```python
from build123d import *

# Parameters (mm, degrees)
SKETCH1_W            = 101.6
SKETCH1_H            = 33.02
BOSS_EXTRUDE1_DEPTH  = 101.6
SKETCH2_W            = 63.5
SKETCH2_H            = 81.28
CUT_EXTRUDE1_DEPTH   = 119.294211186
BOSS_EXTRUDE2_START  = -16.51
BOSS_EXTRUDE2_DEPTH  = 3.81
FILLET2_R            = 2.54
SKETCH4_W            = 12.7
SKETCH4_H            = 12.7
SKETCH4_R            = 1.55
BOSS_EXTRUDE3_DEPTH  = 3.81
FILLET3_R            = 2.54
FILLET2_OF_MIRROR1_R = 2.54


with BuildPart() as part:
    # Sketch1 → Boss-Extrude1 (new body)
    with BuildSketch(Plane.XY):
        Rectangle(SKETCH1_W, SKETCH1_H)
        with BuildLine():
            Line((-31.75, 10.16), (31.75, 10.16))
            ThreePointArc((31.75, 10.16), (41.91, 0), (31.75, -10.16))
            Line((31.75, -10.16), (-31.75, -10.16))
            ThreePointArc((-31.75, -10.16), (-41.91, 0), (-31.75, 10.16))
        make_face(mode=Mode.SUBTRACT)
    extrude(amount=-BOSS_EXTRUDE1_DEPTH)

    # Sketch2 → Cut-Extrude1 (cut, through all)
    with BuildSketch(Plane(origin=(0, 16.51, 0), x_dir=(1, 0, 0), z_dir=(0, 1, 0))):
        with Locations((0, 50.8)):
            Rectangle(SKETCH2_W, SKETCH2_H)
    extrude(amount=-CUT_EXTRUDE1_DEPTH, mode=Mode.SUBTRACT)

    # Sketch3 → Boss-Extrude2 (add, symmetric)
    with BuildSketch(Plane(origin=(0, 16.51, 0), x_dir=(1, 0, 0), z_dir=(0, 1, 0)).offset(BOSS_EXTRUDE2_START)):
        Polygon((-42.926, -4.867948453), (-43.942, -7.195896906), (-42.926, -7.195896906), (-41.91, -4.867948453), (-40.894, -2.54), (-41.91, -2.54), (-41.91, 0), (-43.942, 0), align=None)
    boss_extrude2 = extrude(amount=BOSS_EXTRUDE2_DEPTH, both=True)

    # Fillet2
    fillet2_edges = [part.edges().sort_by_distance(p)[0] for p in [
        (-43.942, 0, 0),
    ]]
    fillet(fillet2_edges, radius=FILLET2_R)

    # Sketch4 → Boss-Extrude3 (add)
    # profile 1 of 4: a face of its own
    with BuildSketch(Plane.XZ.offset(16.51)):
        with Locations((-57.15, -95.25)):
            Rectangle(SKETCH4_W, SKETCH4_H)
        with Locations((-57.15, -95.25)):
            Circle(SKETCH4_R, mode=Mode.SUBTRACT)
    # profile 2 of 4: a face of its own
    with BuildSketch(Plane.XZ.offset(16.51)):
        with Locations((57.15, -95.25)):
            Rectangle(SKETCH4_W, SKETCH4_H)
        with Locations((57.15, -95.25)):
            Circle(SKETCH4_R, mode=Mode.SUBTRACT)
    # profile 3 of 4: a face of its own
    with BuildSketch(Plane.XZ.offset(16.51)):
        with Locations((57.15, -6.35)):
            Rectangle(SKETCH4_W, SKETCH4_H)
        with Locations((57.15, -6.35)):
            Circle(SKETCH4_R, mode=Mode.SUBTRACT)
    # profile 4 of 4: a face of its own
    with BuildSketch(Plane.XZ.offset(16.51)):
        with Locations((-57.15, -6.35)):
            Rectangle(SKETCH4_W, SKETCH4_H)
        with Locations((-57.15, -6.35)):
            Circle(SKETCH4_R, mode=Mode.SUBTRACT)
    extrude(amount=-BOSS_EXTRUDE3_DEPTH)

    # Fillet3
    fillet3_edges = [part.edges().sort_by_distance(p)[0] for p in [
        (-63.5, -12.7, -95.25),
        (-50.8, -12.7, -95.25),
        (63.5, -12.7, -95.25),
        (50.8, -12.7, -95.25),
        (63.5, -12.7, -6.35),
        (50.8, -12.7, -6.35),
        (-63.5, -12.7, -6.35),
        (-50.8, -12.7, -6.35),
    ]]
    fillet(fillet3_edges, radius=FILLET3_R)

    # Mirror1: Boss-Extrude2 across plane
    add(boss_extrude2.mirror(Plane(origin=(0, 0, 0), x_dir=(0, 0, 1), z_dir=(1, 0, 0))))

    # Fillet2 of Mirror1
    fillet2_of_mirror1_edges = [part.edges().sort_by_distance(p)[0] for p in [
        (43.942, 0, 0),
    ]]
    fillet(fillet2_of_mirror1_edges, radius=FILLET2_OF_MIRROR1_R)


solid = part.part
```
Source: CAD feature listing. Evaluate the final solid. Frame: model axes, mm. A direction names the side the tool comes from. Coordinates: 2 decimals unless noted, no trailing zeros. Order: outer loops, then holes, each group sorted by start corner. A loop starts at its lowest first (then second) coordinate and runs counter-clockwise, first axis right, second up. Notation, with made-up numbers: M -10.5,-39 L 10.5,-39 A14 ccw 10.5,-12 Z; hole C 31.25,88.5 d11. An arc over 180 degrees is marked long. Write each question's results on one line, items separated by ' | '. Start each with the question number.
1) Section query D-D (y = -2). Return the cut outline in (x, z).
2) Section query A-A (z = -67). Return the cut outline in (x, y), plus the area to 3 significant figures.
3) Line query: line 1 (Z direction, x = 57.15, y = -15.3); line 2 (X direction, y = -15, z = -95); line 3 (X direction, y = -14, z = -29). Output: solid intervals per line, ascending. Write a range as from..to.
4) Access query for faces 1 (the face through (50.8, 0, -50)), 2 (the face through (-57, -15, -88.9)), 3 (the face through (-50.8, 0, -50)), 4 (the face through (-58.1, -12.7, -4.8)), 5 (the face through (31.75, 13, -50)). Directions: +Z, -Z, +X, -X, +Y, -Y. A direction counts if a zero-diameter tool reaches every point of the face in a straight line with its end or side. Return the directions, or none.
5) Section query B-B (z = -6.35). Return the cut outline in (x, y).
6) Contact query for flat-ended pins moving along their axis: pin 1 Ø3 at (x, y) = (-54, -15) entering from +Z; pin 2 Ø1 at (y, z) = (5, -53) entering from +X; pin 3 Ø2.5 at (x, z) = (-43, 2) entering from -Y. Output: stop coordinate, or through.
7) Draft query along Z for faces 6 (the face through (41.924, 0.053, 4.901)), 7 (the face through (-43, 3.81, 3)), 8 (the face through (-1, -11, -101.6)), 9 (the face through (57, -15, -12.7)). Return one class per face: released by +Z, released by -Z, zero draft, split by the parting line, or undercut.
8) Section query C-C (x = 57.15). Return the cut outline in (y, z), plus the area to 3 significant figures.
Answers:
1) outline: M -50.8,-101.6 L -41.71,-101.6 L -41.71,0 L -41.91,0 L -41.91,2.54 L -40.89,2.54 L -42.93,7.2 L -43.94,7.2 L -42.93,4.87 L -43.52,2.02 A2.54 cw -46.01,0 L -50.8,0 Z; M 40.89,2.54 L 41.91,2.54 L 41.91,0 L 41.71,0 L 41.71,-101.6 L 50.8,-101.6 L 50.8,0 L 46.01,0 A2.54 cw 43.52,2.02 L 42.93,4.87 L 43.94,7.2 L 42.93,7.2 Z
2) outline: M -50.8,-16.51 L -31.75,-16.51 L -31.75,-10.16 A10.16 cw -31.75,10.16 L -31.75,16.51 L -50.8,16.51 Z; M 31.75,-16.51 L 50.8,-16.51 L 50.8,16.51 L 31.75,16.51 L 31.75,10.16 A10.16 cw 31.75,-10.16 Z | area: 934 mm^2
3) line 1: z = -101.6..-96.8, -93.7..-88.9, -12.7..-7.9, -4.8..0 | line 2: x = -63.49..-58.68, -55.62..55.62, 58.68..63.49 | line 3: x = -50.8..-31.75, 31.75..50.8
4) face 1: +X, +Y | face 2: -X, +Y, -Y | face 3: -X, +Y | face 4: +Z, -Z, -X, +Y | face 5: +Y, -Y
5) outline: M -63.5,-16.51 L -58.7,-16.51 L -58.7,-12.7 L -60.96,-12.7 A2.54 ccw -63.5,-15.24 Z; M -55.6,-16.51 L 55.6,-16.51 L 55.6,-12.7 L 53.34,-12.7 A2.54 cw 50.8,-10.16 L 50.8,16.51 L -50.8,16.51 L -50.8,-10.16 A2.54 cw -53.34,-12.7 L -55.6,-12.7 Z; M 58.7,-16.51 L 63.5,-16.51 L 63.5,-15.24 A2.54 ccw 60.96,-12.7 L 58.7,-12.7 Z; hole M -31.75,-10.16 L 31.75,-10.16 A10.16 ccw 31.75,10.16 L -31.75,10.16 A10.16 ccw Z
6) pin 1: stops at z = 0 | pin 2: stops at x = 50.8 | pin 3: stops at y = -3.81
7) face 6: released by +Z | face 7: zero draft | face 8: released by -Z | face 9: undercut
8) outline: M -16.51,-101.6 L -12.7,-101.6 L -12.7,-96.8 L -16.51,-96.8 Z; M -16.51,-93.7 L -12.7,-93.7 L -12.7,-88.9 L -16.51,-88.9 Z; M -16.51,-12.7 L -12.7,-12.7 L -12.7,-7.9 L -16.51,-7.9 Z; M -16.51,-4.8 L -12.7,-4.8 L -12.7,0 L -16.51,0 Z | area: 73.2 mm^2
